Geometry: final body of the model. Coordinates: model frame, mm. Coordinates: 2 decimals unless noted, no trailing zeros. Write each loop counter-clockwise with the first axis right and the second up, starting at its lowest first coordinate (ties: lowest second). Pieces come first, ordered by that corner, then holes.
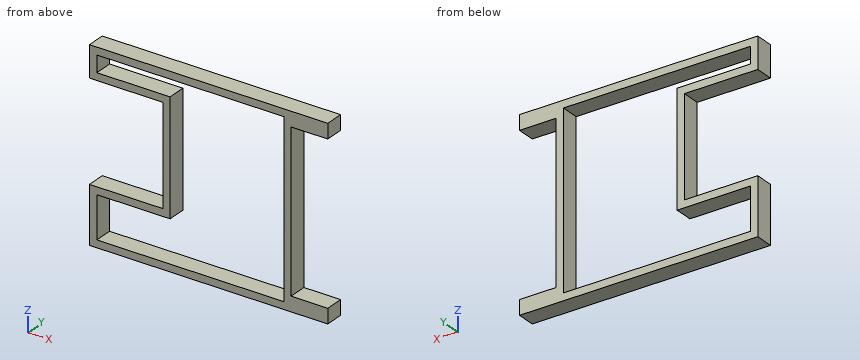
from build123d import *

# Parameters (mm, degrees)
EXTRUDE_4_DEPTH = 5


with BuildPart() as part:
    # 草图1 → 凸台-拉伸4 (new body)
    with BuildSketch(Plane(origin=(0, 0, 0), x_dir=(1, 0, 0), z_dir=(0, 1, 0))):
        Polygon((-44.775072214, 5.646396396), (-24.775072214, 5.646396396), (-24.775072214, -21.353603604), (-44.775072214, -21.353603604), (-44.775072214, -29.853603604), (20.224927786, -29.853603604), (20.224927786, -25.853603604), (10.224927786, -25.853603604), (10.224927786, 17.146396396), (20.224927786, 17.146396396), (20.224927786, 21.146396396), (-44.775072214, 21.146396396), align=None)
        Polygon((-42.775072214, 19.146396396), (8.224927786, 19.146396396), (8.224927786, -27.853603604), (-42.775072214, -27.853603604), (-42.775072214, -23.353603604), (-22.775072214, -23.353603604), (-22.775072214, 7.646396396), (-42.775072214, 7.646396396), align=None, mode=Mode.SUBTRACT)
    extrude(amount=EXTRUDE_4_DEPTH)


solid = part.part
Item 1: Pin query (flat end, axial travel): pin 1 (6 mm diameter, centred on x = -29, z = -1, fed in from +Y); pin 2 (3 mm diameter, centred on y = 1.5, z = -2.5, fed in from +X); pin 3 (1.5 mm diameter, centred on y = 2.5, z = 11.5, fed in from -X). Return the tip coordinate at first contact, or that it passes through.
Derived:
pin 1: passes through
pin 2: stops at x = 10.22
pin 3: stops at x = -24.78
Item 2: Material intervals for probe 1 along Z at (x, y) = (-37.5, 3.1); probe 2 along Z at (x, y) = (17, 2.1); probe 3 along Z at (x, y) = (-20, 1.4), sorted ascending.
Derived:
probe 1: z = -21.15 to -19.15, -7.65 to -5.65, 21.35 to 23.35, 27.85 to 29.85
probe 2: z = -21.15 to -17.15, 25.85 to 29.85
probe 3: z = -21.15 to -19.15, 27.85 to 29.85
Item 3: Section A-A, the plane z = 14. Output: boundary loops of the cut face in (x, y), plus the area to 3 significant figures.
Derived:
outline: (-24.78, 0) - (-22.78, 0) - (-22.78, 5) - (-24.78, 5) - close; (8.22, 0) - (10.22, 0) - (10.22, 5) - (8.22, 5) - close
area: 20.0 mm2
Item 4: Section D-D, the plane x = -39.5. Output: boundary loops of the cut face in (y, z), plus the area to 3 significant figures.
Derived:
outline: (0, -21.15) - (5, -21.15) - (5, -19.15) - (0, -19.15) - close; (0, -7.65) - (5, -7.65) - (5, -5.65) - (0, -5.65) - close; (0, 21.35) - (5, 21.35) - (5, 23.35) - (0, 23.35) - close; (0, 27.85) - (5, 27.85) - (5, 29.85) - (0, 29.85) - close
area: 40.0 mm2
Item 5: Section B-B, the plane x = 7. Output: boundary loops of the cut face in (y, z), plus the area to 3 significant figures.
Derived:
outline: (0, -21.15) - (5, -21.15) - (5, -19.15) - (0, -19.15) - close; (0, 27.85) - (5, 27.85) - (5, 29.85) - (0, 29.85) - close
area: 20.0 mm2
Item 6: Section C-C, the plane y = 1.55. Output: boundary loops of the cut face in (x, z).
Derived:
outline: (-44.78, -21.15) - (20.22, -21.15) - (20.22, -17.15) - (10.22, -17.15) - (10.22, 25.85) - (20.22, 25.85) - (20.22, 29.85) - (-44.78, 29.85) - (-44.78, 21.35) - (-24.78, 21.35) - (-24.78, -5.65) - (-44.78, -5.65) - close; hole (-42.78, -19.15) - (8.22, -19.15) - (8.22, 27.85) - (-42.78, 27.85) - (-42.78, 23.35) - (-22.78, 23.35) - (-22.78, -7.65) - (-42.78, -7.65) - close
